```python
from build123d import *

# Parameters (mm, degrees)
F0_W     = 116.7279371016
F0_H     = 83.6705883693
F0_R     = 5.588
F1_DEPTH = 25.4
F2_DEPTH = 6.35
F3_DEPTH = 25.4


with BuildPart() as f1:
    # F0 (on Front) → F1 (new body)
    with BuildSketch(Plane.XZ):
        with Locations((5.224019289, 15.672063455)):
            Rectangle(F0_W, F0_H)
        with Locations((-33.1561258105, 15.672063455)):
            Circle(F0_R, mode=Mode.SUBTRACT)
        with Locations((30.3438741895, 15.672063455)):
            Circle(F0_R, mode=Mode.SUBTRACT)
        with Locations((-33.1561258105, 15.672063455)):
            Circle(F0_R)
        with Locations((30.3438741895, 15.672063455)):
            Circle(F0_R)
    extrude(amount=F1_DEPTH)

    # F0 (on Front) → F2 (join)
    with BuildSketch(Plane.XZ):
        with Locations((30.3438741895, 15.672063455)):
            Circle(F0_R)
        with Locations((-33.1561258105, 15.672063455)):
            Circle(F0_R)
    extrude(amount=-F2_DEPTH)

    # F3 (add): a face of the model
    f3_faces = [f1.faces().sort_by_distance(p)[0] for p in [
        (-53.1399492618, -12.7, 15.672063455),
    ]]
    extrude(f3_faces, amount=F3_DEPTH)


solid = f1.part
```
Input: part model. Units: mm. Frame: model coordinates. A direction names the side the tool comes from. Give positions to 0.01 mm unless a question says otherwise; leave off trailing zeros. Order: outer loops, then holes, each group sorted by start corner. A loop starts at its lowest first (then second) coordinate and runs counter-clockwise, first axis right, second up. Notation, with made-up numbers: M 72.25,51.5 L 80.25,51.5 A17 ccw 80.25,78.5 Z; hole C 31,59 d10. An arc over 180 degrees is marked long. One line per question, with ' | ' between items.
1) Section C-C on z = 41.5. Output: boundary loops of the cut face in (x, y), and give its area (3 significant figures).
Filled in:
outline: M -78.54,-25.4 L 63.59,-25.4 L 63.59,0 L -78.54,0 Z | area: 3,610 mm2
2) Ray query, L1, parallel to Y at x = -21, z = 50; L2, parallel to Z at x = -33, y = 2.5. Return the intervals inside material, ascending.
Filled in:
L1: y = -25.4 to 0 | L2: z = 10.09 to 21.26
3) Section D-D on x = -49.5. Output: boundary loops of the cut face in (y, z).
Filled in:
outline: M -25.4,-26.16 L 0,-26.16 L 0,57.51 L -25.4,57.51 Z
4) Section A-A on x = 27. Output: boundary loops of the cut face in (y, z).
Filled in:
outline: M -25.4,-26.16 L 0,-26.16 L 0,11.19 L 6.35,11.19 L 6.35,20.15 L 0,20.15 L 0,57.51 L -25.4,57.51 Z
5) Access query for faces 1 (the face through (-6, -13, 57.507)), 2 (the face through (26.225, 3.131, 19.449)). Directions: +Z, -Z, +X, -X, +Y, -Y. A direction counts if a zero-diameter tool reaches every point of the face in a straight line with its end or side. Return the directions, or none.
Filled in:
face 1: +Z, +X, -X, +Y, -Y | face 2: +Y
6) Draft query along X for faces 3 (the face through (63.588, -13, 15)), 4 (the face through (-37.275, 3.131, 19.449)), 5 (the face through (-78.54, -13, 15)). Return one class per face: pulls with the +X half, pulls with the -X half, needs draft (parallel to the pull), parting line crosses it, or undercut.
Filled in:
face 3: pulls with the +X half | face 4: undercut | face 5: pulls with the -X half
7) Contact query for a flat-ended pin moving along its axis: P1, Ø4, axis at x = 0.5, z = -10.5, coming from the +Y side. Output: stop coordinate, or through.
Filled in:
P1: stops at y = 0
8) Section B-B on y = 4.5. Output: boundary loops of the cut face in (x, z).
Filled in:
outline: C -33.16,15.67 d11.18; C 30.34,15.67 d11.18
